Design review of the part built by this model. Coordinates are the model's own, in mm. Face numbers are marked on the shaded views. A direction names the side the tool comes from. Give positions to 0.01 mm unless a question says otherwise; leave off trailing zeros. Write each loop counter-clockwise with the first axis right and the second up, starting at its lowest first coordinate (ties: lowest second). Pieces come first, ordered by that corner, then holes. Notation, with made-up numbers: (13, 33.25) -> (49, 33.25) arc R7 ccw to (49, 44.25) -> close; hole circle Ø8 at (-11, 30). An arc over 180 degrees is marked (long way). Use CSV: the item, a comma, the result in double quotes.
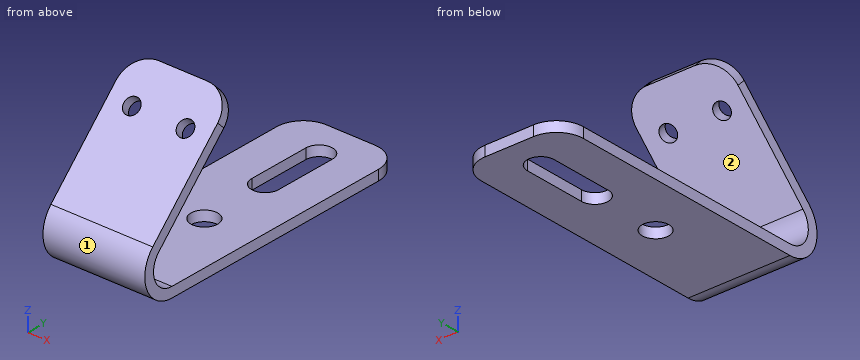
```python
from build123d import *

# Parameters (mm, degrees)
F1_DEPTH = 483.87
F2_R     = 63.5
F3_DEPTH = 48.261
F4_R     = 38.1
F5_DEPTH = 48.26
F7_DEPTH = 48.261
F9_DEPTH = 48.26


with BuildPart() as f1:
    # F0 (on Right) → F1 (new body)
    with BuildSketch(Plane.YZ):
        with BuildLine():
            Line((635, 0), (-635, 0))
            ThreePointArc((-635, 0), (-728.866161, 62.719363), (-706.842049, 173.442049))
            Line((-706.842049, 173.442049), (-257.829243, 622.454855))
            Line((-257.829243, 622.454855), (-291.954216, 656.579828))
            Line((-291.954216, 656.579828), (-740.967022, 207.567022))
            ThreePointArc((-740.967022, 207.567022), (-773.452587, 44.251061), (-635, -48.26))
            Line((-635, -48.26), (635, -48.26))
            Line((635, -48.26), (635, 0))
        make_face()
    extrude(amount=-F1_DEPTH)

    # F2 (on face) → F3 (cut, through all)
    with BuildSketch(Plane.XY):
        with Locations((-238.456383, -177.8)):
            Circle(F2_R)
        with BuildLine():
            Line((-174.956383, 158.261293), (-174.956383, 457.2))
            ThreePointArc((-174.956383, 457.2), (-238.456383, 520.7), (-301.956383, 457.2))
            Line((-301.956383, 457.2), (-301.956383, 158.261293))
            ThreePointArc((-301.956383, 158.261293), (-238.456383, 94.761293), (-174.956383, 158.261293))
        make_face()
    extrude(amount=-F3_DEPTH, mode=Mode.SUBTRACT)

    # F4 (on face) → F5 (cut, through all)
    with BuildSketch(Plane(origin=(0, -474.267022, 474.267022), x_dir=(1, 0, 0), z_dir=(0, -0.707107, 0.707107))):
        with Locations((-369.57, 67.329243)):
            Circle(F4_R)
        with Locations((-114.3, 67.329243)):
            Circle(F4_R)
    extrude(amount=-F5_DEPTH, mode=Mode.SUBTRACT)

    # F6 (on face) → F7 (cut, through all)
    with BuildSketch(Plane.XY):
        with BuildLine():
            ThreePointArc((-127, 635), (-37.197439, 597.802561), (0, 508))
            Line((0, 508), (0, 635))
            Line((0, 635), (-127, 635))
        make_face()
        with BuildLine():
            Line((-483.87, 635), (-483.87, 508))
            ThreePointArc((-483.87, 508), (-446.672561, 597.802561), (-356.87, 635))
            Line((-356.87, 635), (-483.87, 635))
        make_face()
    extrude(amount=-F7_DEPTH, mode=Mode.SUBTRACT)

    # F8 (on face) → F9 (cut, through all)
    with BuildSketch(Plane(origin=(0, -474.267022, 474.267022), x_dir=(1, 0, 0), z_dir=(0, -0.707107, 0.707107))):
        with BuildLine():
            ThreePointArc((-483.87, 130.829243), (-446.672561, 220.631804), (-356.87, 257.829243))
            Line((-356.87, 257.829243), (-483.87, 257.829243))
            Line((-483.87, 257.829243), (-483.87, 130.829243))
        make_face()
        with BuildLine():
            Line((0, 257.829243), (-127, 257.829243))
            ThreePointArc((-127, 257.829243), (-37.197439, 220.631804), (0, 130.829243))
            Line((0, 130.829243), (0, 257.829243))
        make_face()
    extrude(amount=-F9_DEPTH, mode=Mode.SUBTRACT)


solid = f1.part
```
(1) Take a section at B-B (x = -428). Write out the cut boundary in (y, z), then the cut area to 3 significant figures.
Established:
outline,"(-740.97, 207.57) arc R149.86 ccw to (-635, -48.26) -> (613.21, -48.26) -> (613.21, 0) -> (-635, 0) arc R101.6 cw to (-706.84, 173.44) -> (-273.24, 607.05) -> (-307.36, 641.17) -> close"
area,"104,000 mm2"
(2) Take a section at D-D (z = 407). Write out the cut boundary in (x, y).
Established:
outline,"(-483.87, -541.53) -> (0, -541.53) -> (0, -473.28) -> (-483.87, -473.28) -> close"
(3) Take a section at C-C (y = -598). Write out the cut boundary in (x, z).
Established:
outline,"(-483.87, -48.26) -> (0, -48.26) -> (0, 0) -> (-483.87, 0) -> close; (-483.87, 282.28) -> (0, 282.28) -> (0, 350.53) -> (-483.87, 350.53) -> close"
(4) Take a section at A-A (y = -177.8). Write out the cut boundary in (x, z), then the cut area to 3 significant figures.
Established:
outline,"(-483.87, -48.26) -> (-301.96, -48.26) -> (-301.96, 0) -> (-483.87, 0) -> close; (-174.96, -48.26) -> (0, -48.26) -> (0, 0) -> (-174.96, 0) -> close"
area,"17,200 mm2"
(5) Clearance check with flat-ended pins moving along their axes: pin 1 (1.5 mm diameter, centred on x = -83, y = 253, fed in from +Z); pin 2 (1 mm diameter, centred on x = -209, z = 266, fed in from +Y); pin 3 (2 mm diameter, centred on x = -342.5, z = 32, fed in from -Y). State where each tip first meets the part, or that it passes through.
Established:
pin 1,"stops at z = 0"
pin 2,"stops at y = -613.78"
pin 3,"stops at y = -768.24"
(6) For line 1 along X through (y, z) = (-177, -37); line 2 along Z through (x, y) = (-61, -328.5); line 3 along Z through (x, y) = (-455, 293.5), list the stretches that pass through material, from the lowest coordinate up. Write a range as [from, to].
Established:
line 1,"x = [-483.87, -301.95], [-174.96, 0]"
line 2,"z = [-48.26, 0], [551.78, 620.03]"
line 3,"z = [-48.26, 0]"
(7) Tool access review of the marked faces 1 and 2: name each direction out of +Z, -Z, +X, -X, +Y, -Y from which nothing blocks a thin tool from reaching the whole face with its end or side.
Established:
face 1,"+X, -X, -Y"
face 2,"+X, -X, +Y"
